```python
from build123d import *

# Parameters (mm, degrees)
SKETCH1_R                       = 60
BOSS_EXTRUDE1_DEPTH             = 10
SKETCH1_3_R                     = 1.625
CUT_EXTRUDE1_DEPTH              = 86.440037453
CIRPATTERN1_COUNT               = 3
CUT_EXTRUDE2_DEPTH              = 86.440037453
CIRPATTERN2_COUNT               = 3
BOSS_EXTRUDE2_DEPTH             = 77
BOSS_EXTRUDE3_REACH             = 108.685
BOSS_EXTRUDE3_DIRECTION_2_REACH = 108.685
FILLET1_R                       = 15
CUT_EXTRUDE3_DEPTH              = 107.685194831
CUT_EXTRUDE3_DEPTH_BACK         = 107.685194831
SKETCH4_4_R                     = 12.75
BOSS_EXTRUDE4_DEPTH             = 5
BOSS_EXTRUDE4_DEPTH_BACK        = 5
SKETCH7_R                       = 3
CUT_EXTRUDE4_DEPTH              = 135.046990627
SKETCH8_R                       = 3
SKETCH8_R_2                     = 1.625
BOSS_EXTRUDE5_DEPTH             = 10
LPATTERN2_COUNT                 = 2
LPATTERN2_PITCH                 = 32.26
LPATTERN3_COUNT                 = 2
LPATTERN3_PITCH                 = 58.63
FILLET2_R                       = 20
FILLET3_R                       = 20
FILLET4_R                       = 20
FILLET5_R                       = 20
SKETCH9_W                       = 55
SKETCH9_H                       = 7.5
BOSS_EXTRUDE6_DEPTH             = 10
BOSS_EXTRUDE7_DEPTH             = 10
FILLET6_R                       = 20
FILLET7_R                       = 20


with BuildPart() as part:
    # Sketch1 → Boss-Extrude1 (new body)
    with BuildSketch(Plane(origin=(0, 0, 0), x_dir=(1, 0, 0), z_dir=(0, 1, 0))):
        with Locations(Location((0, 0, 0), (0, 0, 270))):
            Circle(SKETCH1_R)
    extrude(amount=BOSS_EXTRUDE1_DEPTH)

    # Sketch1<3> → Cut-Extrude1 (cut, through all)
    with BuildSketch(Plane(origin=(0, 0, 0), x_dir=(1, 0, 0), z_dir=(0, 1, 0))):
        with Locations(Location((0, 50, 0), (0, 0, 270))):
            Circle(SKETCH1_3_R)
    cut_extrude1 = extrude(amount=CUT_EXTRUDE1_DEPTH, mode=Mode.SUBTRACT)

    # CirPattern1: Cut-Extrude1 ×3 about axis
    cirpattern1_axis = Axis((0, 0, 0), (0, 1, 0))
    for i in range(1, CIRPATTERN1_COUNT):
        add(cut_extrude1.rotate(cirpattern1_axis, i * 360 / CIRPATTERN1_COUNT), mode=Mode.SUBTRACT)

    # Sketch2 → Cut-Extrude2 (cut, through all)
    with BuildSketch(Plane(origin=(0, 10, 0), x_dir=(1, 0, 0), z_dir=(0, 1, 0))):
        with BuildLine():
            Line((43.871803017, -40.93), (0, -40.93))
            Line((0, -40.93), (-43.871803017, -40.93))
            ThreePointArc((-43.871803017, -40.93), (0, -60), (43.871803017, -40.93))
        make_face()
    cut_extrude2 = extrude(amount=-CUT_EXTRUDE2_DEPTH, mode=Mode.SUBTRACT)

    # CirPattern2: Cut-Extrude2 ×3 about axis
    cirpattern2_axis = Axis((0, 10.5, 0), (0, -1, 0))
    for i in range(1, CIRPATTERN2_COUNT):
        add(cut_extrude2.rotate(cirpattern2_axis, i * 360 / CIRPATTERN2_COUNT), mode=Mode.SUBTRACT)

    # Sketch3 → Boss-Extrude2 (add)
    with BuildSketch(Plane(origin=(0, 10, 0), x_dir=(1, 0, 0), z_dir=(0, 1, 0))):
        Polygon((-30, -40.93), (0, -40.93), (30, -40.93), (30, -30.93), (-30, -30.93), align=None)
    extrude(amount=-BOSS_EXTRUDE2_DEPTH)

    # Boss-Extrude3: up to this face of the body (flat: up to its plane)
    boss_extrude3_end = Plane(part.part.faces().sort_by_distance((30, -33.5, 35.93))[0])
    # Sketch4 → Boss-Extrude3 (add, up to the picked face)
    with BuildSketch(Plane(origin=(0, 0, 0), x_dir=(0, 0, -1), z_dir=(1, 0, 0)), mode=Mode.PRIVATE) as boss_extrude3_sk1:
        with BuildLine():
            ThreePointArc((-19.02, -19.5), (-22.236059714, -8.072633873), (-30.940100101, 0))
            Line((-30.940100101, 0), (-40.93, 0))
            Line((-40.93, 0), (-40.93, -6.75))
            ThreePointArc((-40.93, -6.75), (-31.91438854, -10.48438854), (-28.18, -19.5))
            ThreePointArc((-28.18, -19.5), (-31.91438854, -28.51561146), (-40.93, -32.25))
            Line((-40.93, -32.25), (-40.93, -41.41))
            ThreePointArc((-40.93, -41.41), (-25.437290424, -34.992709576), (-19.02, -19.5))
        make_face()
    boss_extrude3_tool1 = split(extrude(boss_extrude3_sk1.sketch, amount=BOSS_EXTRUDE3_REACH, mode=Mode.PRIVATE), bisect_by=boss_extrude3_end, keep=Keep.BOTH, mode=Mode.PRIVATE)
    add(boss_extrude3_tool1.solids().sort_by(Axis((0, -10.153116, 31.583116), (1, 0, 0)))[0])

    # Boss-Extrude3 direction 2: up to this face of the body (flat: up to its plane)
    boss_extrude3_direction_2_end = Plane(part.part.faces().sort_by_distance((-30, -33.5, 35.93))[0])
    # Sketch4 → Boss-Extrude3 direction 2 (add, up to the picked face)
    with BuildSketch(Plane(origin=(0, 0, 0), x_dir=(0, 0, -1), z_dir=(1, 0, 0)), mode=Mode.PRIVATE) as boss_extrude3_direction_2_sk1:
        with BuildLine():
            ThreePointArc((-19.02, -19.5), (-22.236059714, -8.072633873), (-30.940100101, 0))
            Line((-30.940100101, 0), (-40.93, 0))
            Line((-40.93, 0), (-40.93, -6.75))
            ThreePointArc((-40.93, -6.75), (-31.91438854, -10.48438854), (-28.18, -19.5))
            ThreePointArc((-28.18, -19.5), (-31.91438854, -28.51561146), (-40.93, -32.25))
            Line((-40.93, -32.25), (-40.93, -41.41))
            ThreePointArc((-40.93, -41.41), (-25.437290424, -34.992709576), (-19.02, -19.5))
        make_face()
    boss_extrude3_direction_2_tool1 = split(extrude(boss_extrude3_direction_2_sk1.sketch, amount=-BOSS_EXTRUDE3_DIRECTION_2_REACH, mode=Mode.PRIVATE), bisect_by=boss_extrude3_direction_2_end, keep=Keep.BOTH, mode=Mode.PRIVATE)
    add(boss_extrude3_direction_2_tool1.solids().sort_by(Axis((0, -10.153116, 31.583116), (-1, 0, 0)))[0])

    # Fillet1
    # the kernel refuses this fillet: 15 mm, written as the material it adds along each edge
    with BuildSketch(Plane(origin=(30, 0, 30.93), x_dir=(0, -0.8200000187317444, -0.5723634940140216), z_dir=(-1, 0, 0))) as fillet1_piece_1:
        with BuildLine():
            CenterArc((27.544705674, -13.254966901), FILLET1_R, 117.912385257, 97.002819116)
            Line((15.244705393, -21.840419312), (14.014705365, -22.698964553))
            Line((14.014705365, -22.698964553), (-1.230000028, -0.858545241))
            Line((-1.230000028, -0.858545241), (-0.858545241, 1.230000028))
            ThreePointArc((-0.858545241, 1.230000028), (0.706809752, 1.32825728), (19.820711794, 1.32549669))
            Line((19.820711794, 1.32549669), (20.522893056, 0))
        make_face()
    extrude(amount=60)
    with BuildSketch(Plane(origin=(30, -0.00517761, 30.93), x_dir=(0, -0.819917344642304, -0.5724819193255918), z_dir=(-1, 0, 0))) as fillet1_piece_2:
        with BuildLine():
            CenterArc((27.542374568, -13.253952614), FILLET1_R, 117.920660394, 97.002819116)
            Line((15.243614398, -21.841181404), (14.013738381, -22.699904283))
            ThreePointArc((14.013738381, -22.699904283), (-1.23412123, -0.861686967), (-0.858722879, 1.229876017))
            Line((-0.858722879, 1.229876017), (0.702372694, 1.325395261))
            ThreePointArc((0.702372694, 1.325395261), (10.259323815, -1.050393215), (19.816274935, 1.325395261))
            Line((19.816274935, 1.325395261), (20.518647629, 0))
        make_face()
    extrude(amount=60)

    # Sketch4<4> → Cut-Extrude3 (cut, two sides: drawn at the far end of the back side and taken through both)
    with BuildSketch(Plane(origin=(0, 0, 0), x_dir=(0, 0, -1), z_dir=(1, 0, 0)).offset(-CUT_EXTRUDE3_DEPTH_BACK)):
        with Locations((-40.93, -19.5)):
            Circle(SKETCH4_4_R)
    extrude(amount=CUT_EXTRUDE3_DEPTH + CUT_EXTRUDE3_DEPTH_BACK, mode=Mode.SUBTRACT)

    # Sketch6 → Boss-Extrude4 (add, two sides: drawn at the far end of the back side and taken through both)
    with BuildSketch(Plane(origin=(0, 0, 0), x_dir=(0, 0, -1), z_dir=(1, 0, 0)).offset(-BOSS_EXTRUDE4_DEPTH_BACK)):
        Polygon((-30.93, -57), (-30.93, -67), (40.93, 0), (30.93, 0), align=None)
    extrude(amount=BOSS_EXTRUDE4_DEPTH + BOSS_EXTRUDE4_DEPTH_BACK)

    # Sketch7 → Cut-Extrude4 (cut, through all)
    with BuildSketch(Plane.XY.offset(40.93)):
        with Locations((-15, -3.375)):
            Circle(SKETCH7_R)
        with Locations((15, -3.375)):
            Circle(SKETCH7_R)
    cut_extrude4 = extrude(amount=-CUT_EXTRUDE4_DEPTH, mode=Mode.SUBTRACT)

    # Sketch8 → Boss-Extrude5 (add)
    # profile 1 of 2: a face of its own
    with BuildSketch(Plane.XY.offset(40.93)):
        with Locations((-15, -3.375)):
            Circle(SKETCH8_R)
        with Locations((-15, -3.375)):
            Circle(SKETCH8_R_2, mode=Mode.SUBTRACT)
    # profile 2 of 2: a face of its own
    with BuildSketch(Plane.XY.offset(40.93)):
        with Locations((15, -3.375)):
            Circle(SKETCH8_R)
        with Locations((15, -3.375)):
            Circle(SKETCH8_R_2, mode=Mode.SUBTRACT)
    boss_extrude5 = extrude(amount=-BOSS_EXTRUDE5_DEPTH)

    # LPattern2: Cut-Extrude4, Boss-Extrude5 ×2
    with Locations(*[(0, -i * LPATTERN2_PITCH, 0) for i in range(1, LPATTERN2_COUNT)]):
        add(cut_extrude4, mode=Mode.SUBTRACT)
        add(boss_extrude5)

    # LPattern3: Cut-Extrude4, Boss-Extrude5 ×2
    with Locations(*[(0, -i * LPATTERN3_PITCH, 0) for i in range(1, LPATTERN3_COUNT)]):
        add(cut_extrude4, mode=Mode.SUBTRACT)
        add(boss_extrude5)

    # Fillet2
    fillet2_edges = [part.edges().sort_by_distance(p)[0] for p in [
        (57.382321286, 5, 17.529095923),
    ]]
    fillet(fillet2_edges, radius=FILLET2_R)

    # Fillet3
    fillet3_edges = [part.edges().sort_by_distance(p)[0] for p in [
        (13.510518268, 5, -58.459095923),
    ]]
    fillet(fillet3_edges, radius=FILLET3_R)

    # Fillet4
    fillet4_edges = [part.edges().sort_by_distance(p)[0] for p in [
        (-13.510518268, 5, -58.459095923),
    ]]
    fillet(fillet4_edges, radius=FILLET4_R)

    # Fillet5
    fillet5_edges = [part.edges().sort_by_distance(p)[0] for p in [
        (-57.382321286, 5, 17.529095923),
    ]]
    fillet(fillet5_edges, radius=FILLET5_R)

    # Sketch9 → Boss-Extrude6 (add)
    with BuildSketch(Plane(origin=(30, 0, 0), x_dir=(0, 0, -1), z_dir=(1, 0, 0))):
        with Locations((-3.43, -63.25)):
            Rectangle(SKETCH9_W, SKETCH9_H)
    boss_extrude6 = extrude(amount=-BOSS_EXTRUDE6_DEPTH)

    # Sketch10 → Boss-Extrude7 (add)
    with BuildSketch(Plane(origin=(30, 0, 0), x_dir=(0, 0, -1), z_dir=(1, 0, 0))):
        Polygon((40.07, -79.25), (40.07, -71.75), (24.07, -59.5), (24.07, -67), align=None)
    boss_extrude7 = extrude(amount=-BOSS_EXTRUDE7_DEPTH)

    # Fillet6
    fillet6_edges = [part.edges().sort_by_distance(p)[0] for p in [
        (25, -59.5, 30.93),
    ]]
    fillet(fillet6_edges, radius=FILLET6_R)

    # Mirror1: Boss-Extrude6, Boss-Extrude7 across plane
    add(boss_extrude6.mirror(Plane(origin=(0, 0, 0), x_dir=(0, 0, 1), z_dir=(1, 0, 0))))
    add(boss_extrude7.mirror(Plane(origin=(0, 0, 0), x_dir=(0, 0, 1), z_dir=(1, 0, 0))))

    # Fillet7
    fillet7_edges = [part.edges().sort_by_distance(p)[0] for p in [
        (-25, -59.5, 30.93),
    ]]
    fillet(fillet7_edges, radius=FILLET7_R)


solid = part.part
```
Read the model definition and answer for the solid it produces. Units are mm, in the model's axes. A direction names the side the tool comes from. Give positions to 0.01 mm unless a question says otherwise; leave off trailing zeros. Loops run counter-clockwise (first coordinate to the right, second up) from the corner with the lowest first, then second, coordinate; pieces in that order, holes last.
Item 1: The part is cut by section A-A (z = -8). Write down the section's boundary in (x, y), and give its area (3 significant figures).
Item 2: For faces 5 (the cylindrical face through (-15.39, -32.66, 28.05)), 6 (the flat face through (25.07, -65.71, -32.18)), 7 (the flat face through (-20.4, -67, 16.1)), 8 (the flat face through (6, -53, 30.93)), 9 (the cylindrical face through (0.42, -5.195, 15.647)), determine the directions among +Z, -Z, +X, -X, +Y, -Y from which every point of the face is accessible in a straight line to the end or side of a thin tool.
Item 3: Find the intervals of material crossed by line 1 along X through (y, z) = (-57, 29); line 2 along Y through (x, z) = (-15, 36); line 3 along X through (y, z) = (7, 25), in increasing order.
Item 4: The mould has two halves that part along X. Classify faces 1 (the cylindrical face through (-24.93, -53.486, 25.227)), 2 (the flat face through (30, -54, 25)), 3 (the cylindrical face through (15.874, -34.265, 36)), 4 (the cylindrical face through (-15.35, -63.59, 36)): released by +X, released by -X, zero draft, split by the parting line, or undercut.
Item 5: Each of these flat-tipped pins is pushed along its axis until it touches: pin 1 Ø5.5 at (x, y) = (15, -35.635) entering from +Z; pin 2 Ø24 at (y, z) = (-28.5, -15.5) entering from -X; pin 3 Ø3 at (x, y) = (-14.5, -4.5) entering from -Z; pin 4 Ø2 at (x, y) = (-26.5, -77) entering from -Z. Where does it stop, or does it pass through?
Taken from the geometry:
1. outline: (-42.64, 0) - (42.64, 0) - (42.64, 10) - (-42.64, 10) - close; (-30, -67) - (-20, -67) - (-20, -59.5) - (-30, -59.5) - close; (-5, -30.7) - (5, -30.7) - (5, -21.13) - (-5, -21.13) - close; (20, -67) - (30, -67) - (30, -59.5) - (20, -59.5) - close
1. area: 1,100 mm2
2. face 5: -Z
2. face 6: -Z, +X, -X
2. face 7: +Z, +X, -X, -Y
2. face 8: none
2. face 9: +X, -X
3. line 1: x = -30 to -20, -5 to 5, 20 to 30
3. line 2: y = -67 to -63.63, -60.38 to -37.26, -34.01 to -31.26, -7.74 to -5, -1.75 to 10
3. line 3: x = -54.27 to -44.93, -41.68 to 41.68, 44.93 to 54.27
4. face 1: zero draft
4. face 2: released by +X
4. face 3: undercut
4. face 4: undercut
5. pin 1: stops at z = 40.93
5. pin 2: stops at x = -5
5. pin 3: stops at z = 30.93
5. pin 4: stops at z = -40.07
